Here's how the part is built. I have some questions about the finished solid (model axes, mm). Give positions to 0.01 mm unless a question says otherwise; leave off trailing zeros. Loops run counter-clockwise (first coordinate to the right, second up) from the corner with the lowest first, then second, coordinate; pieces in that order, holes last. Notation, with made-up numbers: (89.25, 0.25) - (116.25, 0.25) arc R29 cw to (116.25, 35.25) - close; hole circle Ø3 at (41.5, -14). An arc over 180 degrees is marked (long way). Use a Markdown table: item, result.
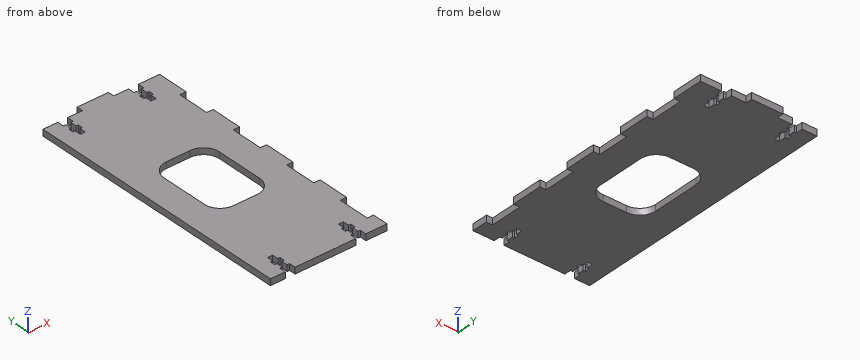
from build123d import *

# Parameters (mm, degrees)
BOSS_EXTRUDE1_DEPTH = 4
CUT_EXTRUDE1_DEPTH  = 96.681816454
SKETCH4_W           = 4
SKETCH4_H           = 19.8
BOSS_EXTRUDE2_DEPTH = 4
SKETCH5_W           = 4
SKETCH5_H           = 10
BOSS_EXTRUDE3_DEPTH = 4
CUT_EXTRUDE2_DEPTH  = 98.212190594


with BuildPart() as part:
    # Sketch1 → Boss-Extrude1 (new body)
    with BuildSketch(Plane.XY):
        Polygon((-9.9, 85), (-9.9, 89), (9.9, 89), (9.9, 85), (34.9, 85), (34.9, -85), (-34.9, -85), (-34.9, 85), align=None)
    extrude(amount=BOSS_EXTRUDE1_DEPTH)

    # Sketch3 → Cut-Extrude1 (cut, through all)
    with BuildSketch(Plane(origin=(0, 0, 0), x_dir=(-1, 0, 0), z_dir=(0, 0, -1))):
        Polygon((25.5, 85), (25.5, 80.9), (24, 80.9), (24, 76.9), (25.4, 76.9), (25.4, 73.9), (24, 73.9), (24, 70), (20.8, 70), (20.8, 73.9), (19.4, 73.9), (19.4, 76.9), (20.8, 76.9), (20.8, 80.9), (19.3, 80.9), (19.3, 85), align=None)
        Polygon((-19.3, 85), (-19.3, 80.9), (-20.8, 80.9), (-20.8, 76.9), (-19.4, 76.9), (-19.4, 73.9), (-20.8, 73.9), (-20.8, 70), (-24, 70), (-24, 73.9), (-25.4, 73.9), (-25.4, 76.9), (-24, 76.9), (-24, 80.9), (-25.5, 80.9), (-25.5, 85), align=None)
        Polygon((-25.5, -85), (-25.5, -80.9), (-24, -80.9), (-24, -76.9), (-25.4, -76.9), (-25.4, -73.9), (-24, -73.9), (-24, -70), (-20.8, -70), (-20.8, -73.9), (-19.4, -73.9), (-19.4, -76.9), (-20.8, -76.9), (-20.8, -80.9), (-19.3, -80.9), (-19.3, -85), align=None)
        Polygon((19.3, -85), (19.3, -80.9), (20.8, -80.9), (20.8, -76.9), (19.4, -76.9), (19.4, -73.9), (20.8, -73.9), (20.8, -70), (24, -70), (24, -73.9), (25.4, -73.9), (25.4, -76.9), (24, -76.9), (24, -80.9), (25.5, -80.9), (25.5, -85), align=None)
    extrude(amount=-CUT_EXTRUDE1_DEPTH, mode=Mode.SUBTRACT)

    # Sketch4 → Boss-Extrude2 (add)
    with BuildSketch(Plane(origin=(0, 0, 0), x_dir=(-1, 0, 0), z_dir=(0, 0, -1))):
        with Locations((-36.9, 35.1)):
            Rectangle(SKETCH4_W, SKETCH4_H)
        with Locations((-36.9, 75.1)):
            Rectangle(SKETCH4_W, SKETCH4_H)
        with Locations((-36.9, -4.9)):
            Rectangle(SKETCH4_W, SKETCH4_H)
        with Locations((-36.9, -44.9)):
            Rectangle(SKETCH4_W, SKETCH4_H)
    extrude(amount=-BOSS_EXTRUDE2_DEPTH)

    # Sketch5 → Boss-Extrude3 (add)
    with BuildSketch(Plane(origin=(0, 0, 0), x_dir=(-1, 0, 0), z_dir=(0, 0, -1))):
        with Locations((-36.9, -80)):
            Rectangle(SKETCH5_W, SKETCH5_H)
    extrude(amount=-BOSS_EXTRUDE3_DEPTH)

    # Sketch6 → Cut-Extrude2 (cut, through all)
    with BuildSketch(Plane(origin=(0, 0, 0), x_dir=(-1, 0, 0), z_dir=(0, 0, -1))):
        with BuildLine():
            Line((-7.5, 25), (7.5, 25))
            ThreePointArc((7.5, 25), (14.571067812, 22.071067812), (17.5, 15))
            Line((17.5, 15), (17.5, -15))
            ThreePointArc((17.5, -15), (14.571067812, -22.071067812), (7.5, -25))
            Line((7.5, -25), (-7.5, -25))
            ThreePointArc((-7.5, -25), (-14.571067812, -22.071067812), (-17.5, -15))
            Line((-17.5, -15), (-17.5, 15))
            ThreePointArc((-17.5, 15), (-14.571067812, 22.071067812), (-7.5, 25))
        make_face()
    extrude(amount=-CUT_EXTRUDE2_DEPTH, mode=Mode.SUBTRACT)


solid = part.part
(1) Suppose I cut it at B-B on x = -12. Write out the boundary of the cut face in (y, z).
A:
| item | result |
|---|---|
| outline | (-85, 0) - (-23.93, 0) - (-23.93, 4) - (-85, 4) - close; (23.93, 0) - (85, 0) - (85, 4) - (23.93, 4) - close |
(2) Will these pins go through, and if not, where does the flat tip stop? pin 1 (2 mm diameter, centred on y = -63.5, z = 3, fed in from +X); pin 2 (0.8 mm diameter, centred on x = 20, z = 2, fed in from +Y); pin 3 (2 mm diameter, centred on x = 37, z = 2, fed in from +Y).
A:
| item | result |
|---|---|
| pin 1 | x = 34.9 |
| pin 2 | y = 80.9 |
| pin 3 | y = 85 |
(3) Suppose I cut it at C-C on y = -64. Write out the boundary of the cut face in (x, z).
A:
| item | result |
|---|---|
| outline | (-34.9, 0) - (34.9, 0) - (34.9, 4) - (-34.9, 4) - close |
(4) Suppose I cut it at A-A on y = -12.5. Write out the boundary of the cut face in (x, z).
A:
| item | result |
|---|---|
| outline | (-34.9, 0) - (-17.5, 0) - (-17.5, 4) - (-34.9, 4) - close; (17.5, 0) - (38.9, 0) - (38.9, 4) - (17.5, 4) - close |
(5) Suppose I cut it at D-D on x = -28.5. Write out the boundary of the cut face in (y, z).
A:
| item | result |
|---|---|
| outline | (-85, 0) - (85, 0) - (85, 4) - (-85, 4) - close |
(6) If I drill on line 1 (X direction, y = 80, z = 2.9); line 2 (X direction, y = 76.5, z = 0.65); line 3 (Y direction, x = -6.5, z = 3.45), over which ranges is the centre line in solid material (lowest first)?
A:
| item | result |
|---|---|
| line 1 | -34.9 to -24, -20.8 to 20.8, 24 to 38.9 |
| line 2 | -34.9 to -25.4, -19.4 to 19.4, 25.4 to 38.9 |
| line 3 | -85 to -25, 25 to 89 |
